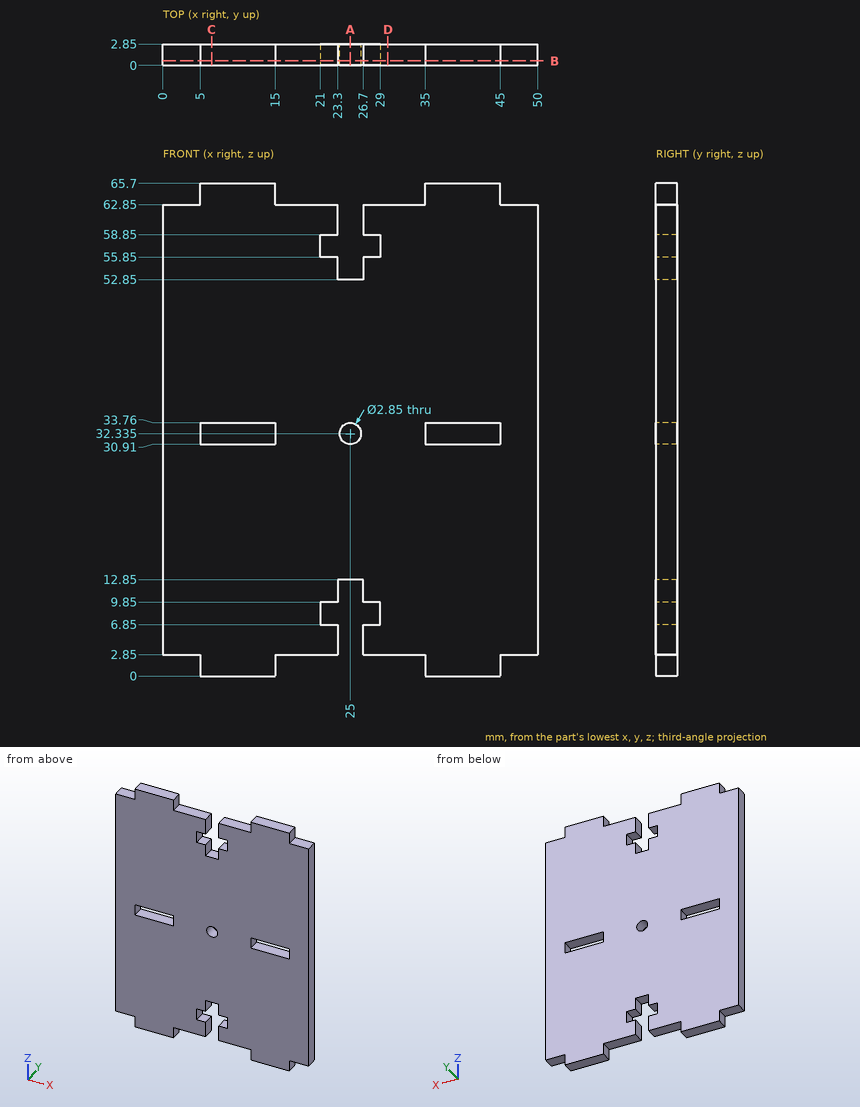
Print and shaded views of the part. All mm, measured from the part's lowest x, y and z. Round coordinates to 2 decimals unless told otherwise and drop trailing zeros. Order: outer loops, then holes, each group sorted by start corner. A loop starts at its lowest first (then second) coordinate and runs counter-clockwise, first axis right, second up.
Q1. Wall check: L1, parallel to Z at x = 5.5, y = 1.8; L2, parallel to X at y = 2.5, z = 58; L3, parallel to X at y = 0.3, z = 11. Give the ranges that are in metal, low to high.
Q2. Slice it at B-B (y = 0.6). State how many separate pieces and enclosed holes the cut face has, and give its area (3 significant figures).
Q3. Slice it at C-C (x = 6.5). Write the cut outline in (y, z), and give its area (3 significant figures).
Q4. Slice it at D-D (x = 30). Write the cut outline in (y, z).
Q5. Slice it at A-A (x = 25). Write the cut outline in (y, z), and give its area (3 significant figures).
Q6. Drop flat-ended pins along their axis: pin 1 (1.4 mm diameter, centred on y = 1, z = 2, fed in from -X); pin 2 (1 mm diameter, centred on x = 18, y = 0.5, fed in from +Z). Give the stop position or say it passes through.
Results below:
1. L1: z = 0 to 30.91, 33.76 to 65.7
1. L2: x = 0 to 21, 29 to 50
1. L3: x = 0 to 23.3, 26.7 to 50
2. separate pieces: 1
2. enclosed holes: 3
2. area: 2,960 mm2
3. outline: (0, 0) - (2.85, 0) - (2.85, 30.91) - (0, 30.91) - close; (0, 33.76) - (2.85, 33.76) - (2.85, 65.7) - (0, 65.7) - close
3. area: 179 mm2
4. outline: (0, 2.85) - (2.85, 2.85) - (2.85, 62.85) - (0, 62.85) - close
5. outline: (0, 12.85) - (2.85, 12.85) - (2.85, 30.91) - (0, 30.91) - close; (0, 33.76) - (2.85, 33.76) - (2.85, 52.85) - (0, 52.85) - close
5. area: 106 mm2
6. pin 1: stops at x = 5
6. pin 2: stops at z = 62.85
